```python
from build123d import *

# Parameters (mm, degrees)
BOSS_EXTRUDE1_DEPTH = 168.275
CUT_EXTRUDE1_DEPTH  = 44.45
FILLET1_R           = 15.24
FILLET2_R           = 76.2
FILLET3_R           = 7.62
FILLET4_R           = 7.62


with BuildPart() as part:
    # Sketch7 → Boss-Extrude1 (new body)
    with BuildSketch(Plane(origin=(0, 0, 0), x_dir=(1, 0, 0), z_dir=(0, 1, 0))):
        Polygon((0, 0), (1016, 0), (1016, -50.8), (927.1, -60.325), (88.9, -60.325), (0, -50.8), align=None)
    extrude(amount=BOSS_EXTRUDE1_DEPTH)

    # Sketch10 → Cut-Extrude1 (cut)
    with BuildSketch(Plane.XZ):
        Polygon((0, 50.8), (0, 25.4), (88.9, 34.925), (927.1, 34.925), (1016, 25.4), (1016, 50.8), (927.1, 60.325), (88.9, 60.325), align=None)
    extrude(amount=-CUT_EXTRUDE1_DEPTH, mode=Mode.SUBTRACT)

    # Fillet1
    fillet1_edges = [part.edges().sort_by_distance(p)[0] for p in [
        (1016, 106.3625, 50.8),
        (0, 106.3625, 50.8),
        (1016, 22.225, 25.4),
        (0, 22.225, 25.4),
    ]]
    fillet(fillet1_edges, radius=FILLET1_R)

    # Fillet2
    fillet2_edges = [part.edges().sort_by_distance(p)[0] for p in [
        (927.1, 106.3625, 60.325),
        (88.9, 106.3625, 60.325),
        (927.1, 22.225, 34.925),
        (88.9, 22.225, 34.925),
    ]]
    fillet(fillet2_edges, radius=FILLET2_R)

    # Fillet3
    fillet3_edges = [part.edges().sort_by_distance(p)[0] for p in [
        (1016, 168.275, 18.552816133),
        (0, 168.275, 18.552816133),
        (49.234552732, 168.275, 56.07513065),
        (3.904199904, 168.275, 47.291761863),
        (1012.095800096, 168.275, 47.291761863),
        (966.765447268, 168.275, 56.07513065),
        (508, 168.275, 60.325),
        (88.905795265, 168.275, 60.216512154),
        (927.094204735, 168.275, 60.216512154),
    ]]
    fillet(fillet3_edges, radius=FILLET3_R)

    # Fillet4
    fillet4_edges = [part.edges().sort_by_distance(p)[0] for p in [
        (1016, 44.45, 18.552816133),
        (0, 44.45, 18.552816133),
        (966.765447268, 44.45, 56.07513065),
        (3.904199904, 44.45, 47.291761863),
        (1012.095800096, 44.45, 47.291761863),
        (508, 44.45, 60.325),
        (49.234552732, 44.45, 56.07513065),
        (88.905795265, 44.45, 60.216512154),
        (927.094204735, 44.45, 60.216512154),
    ]]
    fillet(fillet4_edges, radius=FILLET4_R)


solid = part.part
```
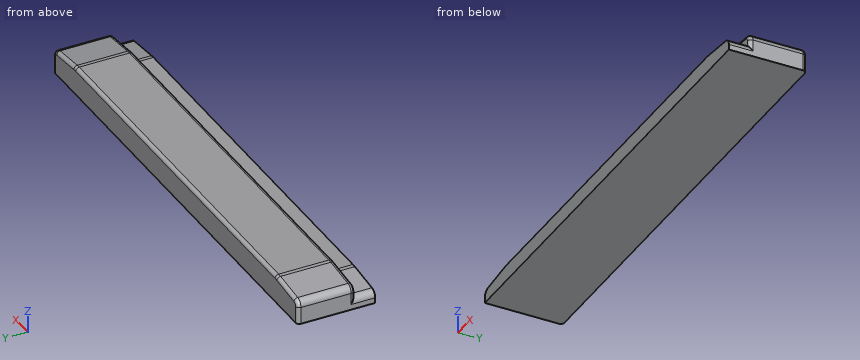
Could you check a few things on this model? Use its own coordinates, in mm. Coordinates: 2 decimals unless noted, no trailing zeros. Order: outer loops, then holes, each group sorted by start corner. A loop starts at its lowest first (then second) coordinate and runs counter-clockwise, first axis right, second up. Notation, with made-up numbers: M -14.5,41 L -4.5,41 A19 ccw -4.5,70 Z; hole C -0.5,10.25 d2. An arc over 180 degrees is marked long. Use one line per item in the form item = value. Start each with the question number.
1. Suppose I cut it at A-A on y = 20. Write out the boundary of the cut face in (x, z) (1 decimal).
2. For pin 1 (22 mm diameter, centred on x = 706, y = 27.5, fed in from +Z) (3 decimals), with a flat end and sliding along its axis, tell me the tip position at first contact or that it passes through.
3. Suppose I cut it at C-C on y = 105. Write out the boundary of the cut face in (x, z) (1 decimal), then the cut area to 3 significant figures.
4. Suppose I cut it at B-B on x = 559.5. Write out the boundary of the cut face in (y, z) (3 decimals), then the cut area to 3 significant figures.
5. Please list where these lines run through material, in increasing order: line 1 (Y direction, x = 641, z = 53); line 2 (Y direction, x = 952, z = 37) (3 decimals); line 3 (Z direction, x = 860, y = 29.5) (3 decimals).
Geometry says:
q1.outline = M 0,0 L 1016,0 L 1016,11.7 A15.2 ccw 1002.4,26.9 L 931.1,34.5 A76.2 ccw 923,34.9 L 93,34.9 A76.2 ccw 84.9,34.5 L 13.6,26.9 A15.2 ccw 0,11.7 Z
q2.pin_1 = 34.925
q3.outline = M 0,0 L 1016,0 L 1016,37.1 A15.2 ccw 1002.4,52.3 L 931.1,59.9 A76.2 ccw 923,60.3 L 93,60.3 A76.2 ccw 84.9,59.9 L 13.6,52.3 A15.2 ccw 0,37.1 Z
q3.area = 60,400 mm^2
q4.outline = M 0,0 L 168.275,0 L 168.275,52.705 A7.62 ccw 160.655,60.325 L 52.07,60.325 A7.62 ccw 44.45,52.705 L 44.45,34.925 L 0,34.925 Z
q4.area = 9,000 mm^2
q5.line_1 = 44.46 to 168.27
q5.line_2 = 44.45 to 168.275
q5.line_3 = 0 to 34.925
